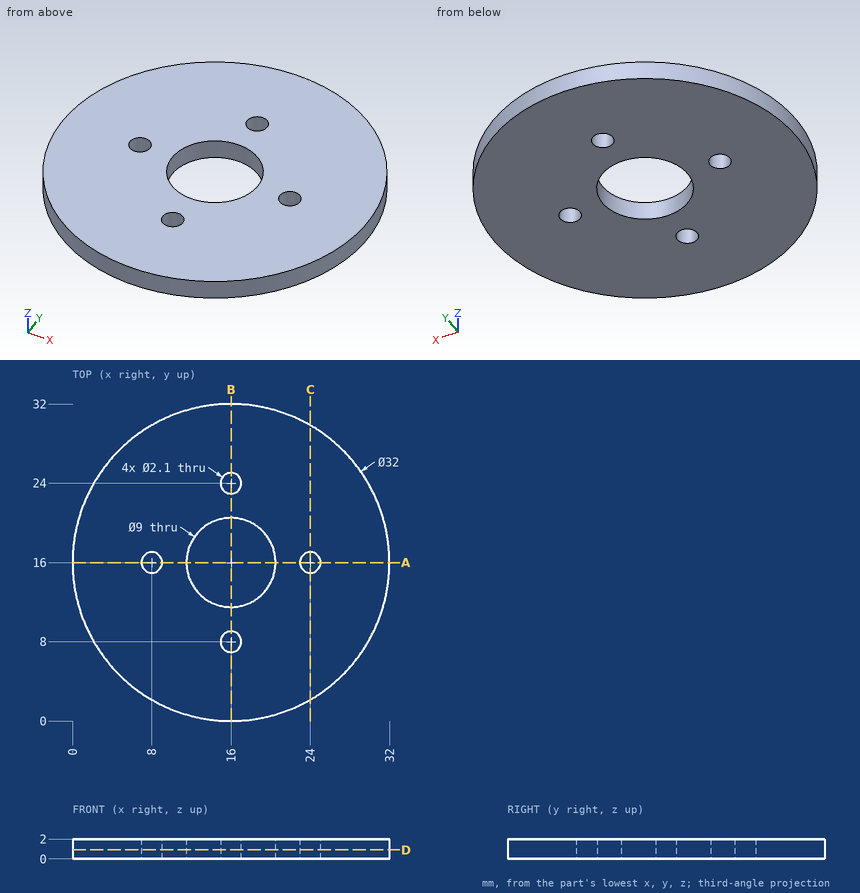
Part print with two shaded views. Sizes in mm from the minimum x, y, z corner. Round coordinates to 2 decimals unless told otherwise and drop trailing zeros. Loops run counter-clockwise (first coordinate to the right, second up) from the corner with the lowest first, then second, coordinate; pieces in that order, holes last. Notation, with made-up numbers: M -39.75,8 L -24.75,8 A25 ccw -24.75,34 Z; hole C 46,62.5 d6. An arc over 180 degrees is marked long. Put each result on its own line as item: value. Start each with the question number.
Item 1: Drill centre lines: line 1 along Y through (x, z) = (16, 0.9); line 2 along X through (y, z) = (15.5, 1.6); line 3 along Y through (x, z) = (18, 1). Where is each one in solid material? Low to high.
Item 2: Cut at C-C (x = 24). List the corners of the cut face in (y, z), then the cut area to 3 significant figures.
Item 3: Cut at D-D (z = 0.9). List the corners of the cut face in (x, y), then the cut area to 3 significant figures.
Item 4: Cut at A-A (y = 16). List the corners of the cut face in (x, z), then the cut area to 3 significant figures.
Answer block:
1. line 1: 0 to 6.95, 9.05 to 11.5, 20.5 to 22.95, 25.05 to 32
1. line 2: 0.01 to 7.08, 8.92 to 11.53, 20.47 to 23.08, 24.92 to 31.99
1. line 3: 0.13 to 11.97, 20.03 to 31.87
2. outline: M 2.14,0 L 14.95,0 L 14.95,2 L 2.14,2 Z; M 17.05,0 L 29.86,0 L 29.86,2 L 17.05,2 Z
2. area: 51.2 mm2
3. outline: C 16,16 d32; hole C 8,16 d2.1; hole C 16,16 d9; hole C 16,8 d2.1; hole C 16,24 d2.1; hole C 24,16 d2.1
3. area: 727 mm2
4. outline: M 0,0 L 6.95,0 L 6.95,2 L 0,2 Z; M 9.05,0 L 11.5,0 L 11.5,2 L 9.05,2 Z; M 20.5,0 L 22.95,0 L 22.95,2 L 20.5,2 Z; M 25.05,0 L 32,0 L 32,2 L 25.05,2 Z
4. area: 37.6 mm2
